Read the model definition and answer for the solid it produces. Units are mm, in the model's axes. A direction names the side the tool comes from. Coordinates: 2 decimals unless noted, no trailing zeros. Write each loop counter-clockwise with the first axis right and the second up, starting at its lowest first coordinate (ties: lowest second). Pieces come first, ordered by that corner, then holes. Notation, with made-up numbers: (4, -25.75) -> (43, -25.75) arc R19 ccw to (43, 3.25) -> close; hole circle Ø2 at (-15, 42.25). An arc over 180 degrees is marked (long way). One line per item, written item: value. Start each with the question number.
1. Find section A-A, the plane x = 0. Write down the section's boundary in (y, z), and give its area (3 significant figures).
2. Find section C-C, the plane y = 1.15. Write down the section's boundary in (x, z) (1 decimal), and give its area (3 significant figures).
3. Consider line 1 along X through (y, z) = (0.55, 0); line 2 along Y through (x, z) = (-1.25, -4); line 3 along X through (y, z) = (0.85, 0). Determine where each line is inside the solid, lowest interval first.
4. Find section D-D, the plane y = -2.2. Write down the section's boundary in (x, z).
5. Given P1, Ø3, axis at x = 0.5, y = 1, coming from the +Z side; P2, Ø1, axis at x = -2, y = -1.5, coming from the -Z side; P3, Ø3, axis at x = 3, y = -2, coming from the +Z side; P4, Ø1, axis at y = 1, z = 1.5, coming from the +X side, each flat-ended and moving along its own axis, determine where each tip first touches the part or whether it passes through.
6. For faces 4 (the cylindrical face through (-3.874, -0.011, -0.86)), 5 (the cylindrical face through (4.685, -1.146, 2.987)), 6 (the cylindrical face through (-1.45, 0.04, -1.89)), determine the directions among +Z, -Z, +X, -X, +Y, -Y from which every point of the face is accessible in a straight line to the end or side of a thin tool.
7. For a pull along Y with two mould halves and no side action, classify faces 1 (the flat face through (-2, -2.778, 2)), 2 (the flat face through (-4, -0.794, -1)), 3 (the flat face through (-3, 2.778, 0)) as pulls with the +Y half, pulls with the -Y half, needs draft (parallel to the pull), parting line crosses it, or undercut.
8. Find section B-B, the plane z = 0. Write down the section's boundary in (x, y).
```python
from build123d import *

# Parameters (mm, degrees)
SKETCH1_R           = 5.55625
BOSS_EXTRUDE1_DEPTH = 2.778125
SKETCH2_R           = 7.9375
BOSS_EXTRUDE2_DEPTH = 2.54
SKETCH3_R           = 8.070808391
SKETCH3_R_2         = 3.96875
CUT_EXTRUDE1_DEPTH  = 0.79375
SKETCH4_R           = 2.38125
CUT_EXTRUDE2_DEPTH  = 13.525163734
FILLET1_R           = 1.27


with BuildPart() as part:
    # Sketch1 → Boss-Extrude1 (new, symmetric)
    with BuildSketch(Plane(origin=(0, 0, 0), x_dir=(1, 0, 0), z_dir=(0, 1, 0))):
        with Locations(Location((0, 0, 0), (0, 0, 270))):
            Circle(SKETCH1_R)
    extrude(amount=BOSS_EXTRUDE1_DEPTH, both=True)

    # Sketch2 → Boss-Extrude2 (add)
    with BuildSketch(Plane(origin=(0, 2.778125, 0), x_dir=(1, 0, 0), z_dir=(0, 1, 0))):
        with Locations(Location((0, 0, 0), (0, 0, 270))):
            Circle(SKETCH2_R)
    extrude(amount=-BOSS_EXTRUDE2_DEPTH)

    # Sketch3 → Cut-Extrude1 (cut, symmetric)
    with BuildSketch(Plane(origin=(0, 0, 0), x_dir=(1, 0, 0), z_dir=(0, 1, 0))):
        Circle(SKETCH3_R)
        with Locations(Location((0, 0, 0), (0, 0, 270))):
            Circle(SKETCH3_R_2, mode=Mode.SUBTRACT)
    extrude(amount=CUT_EXTRUDE1_DEPTH, both=True, mode=Mode.SUBTRACT)

    # Sketch4 → Cut-Extrude2 (cut, through all)
    with BuildSketch(Plane(origin=(0, 2.778125, 0), x_dir=(1, 0, 0), z_dir=(0, 1, 0))):
        with Locations(Location((0, 0, 0), (0, 0, 270))):
            Circle(SKETCH4_R)
    extrude(amount=-CUT_EXTRUDE2_DEPTH, mode=Mode.SUBTRACT)

    # Fillet1
    fillet1_edges = [part.edges().sort_by_distance(p)[0] for p in [
        (0, -2.778125, -5.55625),
        (0, 2.778125, -7.9375),
    ]]
    fillet(fillet1_edges, radius=FILLET1_R)


solid = part.part
```
Answer block:
1. outline: (-2.78, -4.29) arc R1.27 ccw to (-1.51, -5.56) -> (-0.79, -5.56) -> (-0.79, -3.97) -> (0.79, -3.97) -> (0.79, -7.94) -> (1.51, -7.94) arc R1.27 ccw to (2.78, -6.67) -> (2.78, -2.38) -> (-2.78, -2.38) -> close; (-2.78, 2.38) -> (2.78, 2.38) -> (2.78, 6.67) arc R1.27 ccw to (1.51, 7.94) -> (0.79, 7.94) -> (0.79, 3.97) -> (-0.79, 3.97) -> (-0.79, 5.56) -> (-1.51, 5.56) arc R1.27 ccw to (-2.78, 4.29) -> close
1. area: 38.3 mm2
2. outline: circle Ø15.9 at (0, 0); hole circle Ø4.8 at (0, 0)
2. area: 180 mm2
3. line 1: x = -3.97 to -2.38, 2.38 to 3.97
3. line 2: y = -2.78 to -0.79, 0.79 to 2.78
3. line 3: x = -7.94 to -2.38, 2.38 to 7.94
4. outline: circle Ø10.7 at (0, 0); hole circle Ø4.76 at (0, 0)
5. P1: stops at z = 7.94
5. P2: stops at z = -5.35
5. P3: stops at z = 5.33
5. P4: stops at x = 7.87
6. face 4: none
6. face 5: -Y
6. face 6: +Y, -Y
7. face 1: pulls with the -Y half
7. face 2: undercut
7. face 3: pulls with the +Y half
8. outline: (-7.94, 0.79) -> (-3.97, 0.79) -> (-3.97, -0.79) -> (-5.56, -0.79) -> (-5.56, -1.51) arc R1.27 ccw to (-4.29, -2.78) -> (-2.38, -2.78) -> (-2.38, 2.78) -> (-6.67, 2.78) arc R1.27 ccw to (-7.94, 1.51) -> close; (2.38, -2.78) -> (4.29, -2.78) arc R1.27 ccw to (5.56, -1.51) -> (5.56, -0.79) -> (3.97, -0.79) -> (3.97, 0.79) -> (7.94, 0.79) -> (7.94, 1.51) arc R1.27 ccw to (6.67, 2.78) -> (2.38, 2.78) -> close
